Could you check a few things on this model? Use its own coordinates, in mm. A direction names the side the tool comes from. Round coordinates to 2 decimals unless told otherwise and drop trailing zeros. Loops run counter-clockwise (first coordinate to the right, second up) from the corner with the lowest first, then second, coordinate; pieces in that order, holes last. Notation, with made-up numbers: (40.5, 2) - (62.5, 2) arc R28 cw to (62.5, 36) - close; hole circle Ø1 at (-8.75, -29). An arc over 180 degrees is marked (long way). Use one line per item in the form item = value.
```python
from build123d import *

# Parameters (mm, degrees)
SKETCH_1_R      = 6
SKETCH_1_R_2    = 4.75
EXTRUDE_1_DEPTH = 12
SKETCH_2_R      = 5.5
EXTRUDE_2_DEPTH = 2
SKETCH_3_R      = 2.75
EXTRUDE_3_DEPTH = 8


with BuildPart() as part:
    # 草图1 → 凸台-拉伸1 (new body)
    with BuildSketch(Plane(origin=(0, 0, 0), x_dir=(1, 0, 0), z_dir=(0, 1, 0))):
        with Locations(Location((0, 0, 0), (0, 0, 270))):
            Circle(SKETCH_1_R)
        with Locations(Location((0, 0, 0), (0, 0, 270))):
            Circle(SKETCH_1_R_2, mode=Mode.SUBTRACT)
    extrude(amount=EXTRUDE_1_DEPTH)

    # 草图2 → 凸台-拉伸2 (add)
    with BuildSketch(Plane(origin=(0, 12, 0), x_dir=(1, 0, 0), z_dir=(0, 1, 0))):
        with Locations(Location((0, 0, 0), (0, 0, 270))):
            Circle(SKETCH_2_R)
    extrude(amount=EXTRUDE_2_DEPTH)

    # 草图3 → 凸台-拉伸3 (add)
    with BuildSketch(Plane(origin=(0, 14, 0), x_dir=(1, 0, 0), z_dir=(0, 1, 0))):
        with Locations(Location((0, 0, 0), (0, 0, 270))):
            Circle(SKETCH_3_R)
    extrude(amount=EXTRUDE_3_DEPTH)


solid = part.part
```
1. If we section it at C-C, the plane y = 7.75: Write out the boundary of the cut face in (x, z).
Solution:
outline = circle Ø12 at (0, 0); hole circle Ø9.5 at (0, 0)
2. Please list where these lines run through material, in increasing order: line 1 along X through (y, z) = (5.25, 0); line 2 along Y through (x, z) = (-2.25, 3.75); line 3 along Y through (x, z) = (-1, 1).
Solution:
line_1 = -6 to -4.75, 4.75 to 6
line_2 = 12 to 14
line_3 = 12 to 22
3. On a 3-axis mill with a long thin cutter (end or side, diameter ignored), from which of +Z, -Z, +X, -X, +Y, -Y can I reach the whole of each face in a straight line? I mean faces 4 (the face through (-2.89, 5.92, -3.77)), 5 (the face through (-5, 12, 3)), 6 (the face through (1.802, 5.916, 5.723)). Say none if no direction works.
Solution:
face_4 = -Y
face_5 = +Y
face_6 = +Y, -Y
4. We'd pull the mould along X, two halves only. Please class faces 1 (the face through (0, 12, 0)), 2 (the face through (-2.685, 17.944, -0.596)), 3 (the face through (3, 14, 1)): +X half, -X half, draft (parallel to the pull), parting line (faces both ways), or undercut.
Solution:
face_1 = undercut
face_2 = parting line
face_3 = draft
5. If we section it at A-A, the plane z = 0: Write out the boundary of the cut face in (x, y), plus the area to 3 significant figures.
Solution:
outline = (-6, 0) - (-4.75, 0) - (-4.75, 12) - (4.75, 12) - (4.75, 0) - (6, 0) - (6, 12) - (5.5, 12) - (5.5, 14) - (2.75, 14) - (2.75, 22) - (-2.75, 22) - (-2.75, 14) - (-5.5, 14) - (-5.5, 12) - (-6, 12) - close
area = 96.0 mm^2
6. For P1, Ø2, axis at y = 11.5, z = -4.5, coming from the +X side; P2, Ø1.5, axis at x = -1.5, z = 4.5, coming from the -Y side; P3, Ø4, axis at y = 17.5, z = 3.5, coming from the -X side; P4, Ø4, axis at y = 12, z = 4.5, coming from the +X side, each with a flat end and sliding along its axis, tell me the tip position at first contact or that it passes through.
Solution:
P1 = 4.87
P2 = 0
P3 = -2.3
P4 = 5.45
7. If we section it at B-B, the plane x = 0: Write out the boundary of the cut face in (y, z), plus the area to 3 significant figures.
Solution:
outline = (0, -6) - (12, -6) - (12, -5.5) - (14, -5.5) - (14, -2.75) - (22, -2.75) - (22, 2.75) - (14, 2.75) - (14, 5.5) - (12, 5.5) - (12, 6) - (0, 6) - (0, 4.75) - (12, 4.75) - (12, -4.75) - (0, -4.75) - close
area = 96.0 mm^2
8. If we section it at D-D, the plane y = 15.75: Write out the boundary of the cut face in (x, z).
Solution:
outline = circle Ø5.5 at (0, 0)
